from build123d import *

# Parameters (mm, degrees)
CROQUIS1_W              = 58
CROQUIS1_H              = 95
SALIENTE_EXTRUIR4_DEPTH = 1
CROQUIS3_W              = 58
CROQUIS3_H              = 62
SALIENTE_EXTRUIR5_DEPTH = 1
CROQUIS4_W              = 58
CROQUIS4_H              = 62
SALIENTE_EXTRUIR6_DEPTH = 1
CORTAR_EXTRUIR4_DEPTH   = 1
CORTAR_EXTRUIR5_DEPTH   = 1
CROQUIS8_R              = 2.5
CORTAR_EXTRUIR6_DEPTH   = 1
CORTAR_EXTRUIR7_START   = -1
CROQUIS9_R              = 2.5
CORTAR_EXTRUIR7_DEPTH   = 1
CROQUIS10_R             = 2
CORTAR_EXTRUIR8_DEPTH   = 1
CROQUIS11_R             = 2
CORTAR_EXTRUIR9_DEPTH   = 1


with BuildPart() as part:
    # Croquis1 → Saliente-Extruir4 (new body)
    with BuildSketch(Plane(origin=(0, 0, 0), x_dir=(1, 0, 0), z_dir=(0, 1, 0))):
        Rectangle(CROQUIS1_W, CROQUIS1_H)
    extrude(amount=SALIENTE_EXTRUIR4_DEPTH)

    # Croquis3 → Saliente-Extruir5 (add)
    with BuildSketch(Plane.XY.offset(47.5)):
        with Locations((0, 32)):
            Rectangle(CROQUIS3_W, CROQUIS3_H)
    extrude(amount=-SALIENTE_EXTRUIR5_DEPTH)

    # Croquis4 → Saliente-Extruir6 (add)
    with BuildSketch(Plane(origin=(0, 0, -47.5), x_dir=(-1, 0, 0), z_dir=(0, 0, -1))):
        with Locations((0, 32)):
            Rectangle(CROQUIS4_W, CROQUIS4_H)
    extrude(amount=-SALIENTE_EXTRUIR6_DEPTH)

    # Croquis6 → Cortar-Extruir4 (cut)
    with BuildSketch(Plane(origin=(0, 0, -47.5), x_dir=(-1, 0, 0), z_dir=(0, 0, -1))):
        Polygon((1, 63), (29, 10), (29, 63), align=None)
    extrude(amount=-CORTAR_EXTRUIR4_DEPTH, mode=Mode.SUBTRACT)

    # Croquis7 → Cortar-Extruir5 (cut)
    with BuildSketch(Plane.XY.offset(47.5)):
        Polygon((-1, 63), (-29, 10), (-29, 63), align=None)
    extrude(amount=-CORTAR_EXTRUIR5_DEPTH, mode=Mode.SUBTRACT)

    # Croquis8 → Cortar-Extruir6 (cut)
    with BuildSketch(Plane.XY.offset(47.5)):
        with Locations((14, 48)):
            Circle(CROQUIS8_R)
    extrude(amount=-CORTAR_EXTRUIR6_DEPTH, mode=Mode.SUBTRACT)

    # Croquis9 → Cortar-Extruir7 (cut)
    with BuildSketch(Plane(origin=(0, 0, -47.5), x_dir=(-1, 0, 0), z_dir=(0, 0, -1)).offset(CORTAR_EXTRUIR7_START)):
        with Locations(Location((-14, 48, 0), (0, 0, 180))):
            Circle(CROQUIS9_R)
    extrude(amount=CORTAR_EXTRUIR7_DEPTH, mode=Mode.SUBTRACT)

    # Croquis10 → Cortar-Extruir8 (cut)
    with BuildSketch(Plane.XY.offset(47.5)):
        with Locations((-4.910218483, 43.157065968)):
            Circle(CROQUIS10_R)
        with Locations((2.184940403, 23.167473614)):
            Circle(CROQUIS10_R)
        with Locations((22.174532757, 30.267910044)):
            Circle(CROQUIS10_R)
    extrude(amount=-CORTAR_EXTRUIR8_DEPTH, mode=Mode.SUBTRACT)

    # Croquis11 → Cortar-Extruir9 (cut)
    with BuildSketch(Plane(origin=(0, 1, 0), x_dir=(1, 0, 0), z_dir=(0, 1, 0))):
        with Locations(Location((-19, 36.5, 0), (0, 0, 270))):
            Circle(CROQUIS11_R)
        with Locations(Location((19, 36.5, 0), (0, 0, 90))):
            Circle(CROQUIS11_R)
        with Locations(Location((19, -36.5, 0), (0, 0, 270))):
            Circle(CROQUIS11_R)
        with Locations(Location((-19, -36.5, 0), (0, 0, 90))):
            Circle(CROQUIS11_R)
    extrude(amount=-CORTAR_EXTRUIR9_DEPTH, mode=Mode.SUBTRACT)


solid = part.part
Input: part model. Units: mm. Frame: model coordinates. A direction names the side the tool comes from. Round coordinates to 2 decimals unless told otherwise and drop trailing zeros. Order: outer loops, then holes, each group sorted by start corner. A loop starts at its lowest first (then second) coordinate and runs counter-clockwise, first axis right, second up.
1. Cut plane A-A, the plane x = 14. Output: boundary loops of the cut face in (y, z), then the cut area to 3 significant figures.
The answers:
outline: (0, -47.5) - (45.5, -47.5) - (45.5, -46.5) - (1, -46.5) - (1, 46.5) - (45.5, 46.5) - (45.5, 47.5) - (0, 47.5) - close; (50.5, -47.5) - (63, -47.5) - (63, -46.5) - (50.5, -46.5) - close; (50.5, 46.5) - (63, 46.5) - (63, 47.5) - (50.5, 47.5) - close
area: 209 mm2
2. Cut plane C-C, the plane y = 12.5. Output: boundary loops of the cut face in (x, z).
The answers:
outline: (-27.68, -47.5) - (29, -47.5) - (29, -46.5) - (-27.68, -46.5) - close; (-27.68, 46.5) - (29, 46.5) - (29, 47.5) - (-27.68, 47.5) - close
3. Mould query, pull axis X, two halves, no side actions, for faces 4 (the face through (1.92, 25.15, 47.01)), 5 (the face through (6, 25, 47.5)), 6 (the face through (-14.804, 36.871, 47.007)), 7 (the face through (20.983, 0.507, 36.24)). Classes: released by +X, released by -X, zero draft, split by the parting line, or undercut.
The answers:
face 4: undercut
face 5: zero draft
face 6: released by -X
face 7: undercut
4. Material intervals for line 1 (X direction, y = 0.45, z = 36.5); line 2 (Z direction, x = 15, y = 17.5); line 3 (Y direction, x = -16.5, z = -6.5), sorted ascending.
The answers:
line 1: x = -29 to -21, -17 to 17, 21 to 29
line 2: z = -47.5 to -46.5, 46.5 to 47.5
line 3: y = 0 to 1
5. Cut plane B-B, the plane z = -36.5. Output: boundary loops of the cut face in (x, y), then the cut area to 3 significant figures.
The answers:
outline: (-29, 0) - (-21, 0) - (-21, 1) - (-29, 1) - close; (-17, 0) - (17, 0) - (17, 1) - (-17, 1) - close; (21, 0) - (29, 0) - (29, 1) - (21, 1) - close
area: 50.0 mm2
6. Pin query (flat end, axial travel): P1, Ø3.5, axis at x = 22.17, y = 30.27, coming from the +Z side; P2, Ø6.5, axis at x = -19, z = 36.5, coming from the +Y side. Return the tip coordinate at first contact, or that it passes through.
The answers:
P1: stops at z = -46.5
P2: stops at y = 1
7. Set-up query: faces 1 (the face through (-20.983, 0.507, 36.76)), 2 (the face through (0, 1, -1)), 3 (the face through (20.59, 29.05, 47.01)). Return all of +Z, -Z, +X, -X, +Y, -Y with unobstructed straight access to the full face (end or side cutting, diameter ignored); none if empty.
The answers:
face 1: +Y, -Y
face 2: +X, -X, +Y
face 3: +Z
8. Cut plane D-D, the plane y = 48. Output: boundary loops of the cut face in (x, z).
The answers:
outline: (-8.92, -47.5) - (11.5, -47.5) - (11.5, -46.5) - (-8.92, -46.5) - close; (-8.92, 46.5) - (11.5, 46.5) - (11.5, 47.5) - (-8.92, 47.5) - close; (16.5, -47.5) - (29, -47.5) - (29, -46.5) - (16.5, -46.5) - close; (16.5, 46.5) - (29, 46.5) - (29, 47.5) - (16.5, 47.5) - close
